Read the model definition and answer for the solid it produces. Units are mm, in the model's axes. Face numbers are marked on the shaded views. A direction names the side the tool comes from. Coordinates: 2 decimals unless noted, no trailing zeros. Loops run counter-clockwise (first coordinate to the right, second up) from the corner with the lowest first, then second, coordinate; pieces in that order, holes last.
from build123d import *

# Parameters (mm, degrees)
F0_R     = 12.7
F1_DEPTH = 25.4
F2_R     = 12.7
F3_DEPTH = 3.175
F5_DEPTH = 25.4


with BuildPart() as f1:
    # F0 (on Top) → F1 (new body)
    with BuildSketch(Plane.XY):
        Circle(F0_R)
        with BuildLine():
            ThreePointArc((8.614346, 1.798068), (8.753463, 0.903814), (8.8, 0))
            ThreePointArc((8.8, 0), (8.753463, -0.903814), (8.614346, -1.798068))
            Line((8.614346, -1.798068), (10.468267, -2.86843))
            Line((10.468267, -2.86843), (7.718267, -7.63157))
            Line((7.718267, -7.63157), (5.864346, -6.561208))
            ThreePointArc((5.864346, -6.561208), (4.4, -7.621024), (2.75, -8.359276))
            Line((2.75, -8.359276), (2.75, -10.5))
            Line((2.75, -10.5), (-2.75, -10.5))
            Line((-2.75, -10.5), (-2.75, -8.359276))
            ThreePointArc((-2.75, -8.359276), (-4.4, -7.621024), (-5.864346, -6.561208))
            Line((-5.864346, -6.561208), (-7.718267, -7.63157))
            Line((-7.718267, -7.63157), (-10.468267, -2.86843))
            Line((-10.468267, -2.86843), (-8.614346, -1.798068))
            ThreePointArc((-8.614346, -1.798068), (-8.8, 0), (-8.614346, 1.798068))
            Line((-8.614346, 1.798068), (-10.468267, 2.86843))
            Line((-10.468267, 2.86843), (-7.718267, 7.63157))
            Line((-7.718267, 7.63157), (-5.864346, 6.561208))
            ThreePointArc((-5.864346, 6.561208), (-4.4, 7.621024), (-2.75, 8.359276))
            Line((-2.75, 8.359276), (-2.75, 10.5))
            Line((-2.75, 10.5), (2.75, 10.5))
            Line((2.75, 10.5), (2.75, 8.359276))
            ThreePointArc((2.75, 8.359276), (4.4, 7.621024), (5.864346, 6.561208))
            Line((5.864346, 6.561208), (7.718267, 7.63157))
            Line((7.718267, 7.63157), (10.468267, 2.86843))
            Line((10.468267, 2.86843), (8.614346, 1.798068))
        make_face(mode=Mode.SUBTRACT)
    extrude(amount=F1_DEPTH)

    # F2 (on face) → F3 (join)
    with BuildSketch(Plane.XY.offset(25.4)):
        Circle(F2_R)
    extrude(amount=F3_DEPTH)

    # F4 (on face) → F5 (join)
    with BuildSketch(Plane.XY.offset(28.575)):
        Polygon((3.666174, 6.35), (-3.666174, 6.35), (-7.332348, 0), (-3.666174, -6.35), (3.666174, -6.35), (7.332348, 0), align=None)
    extrude(amount=F5_DEPTH)


solid = f1.part
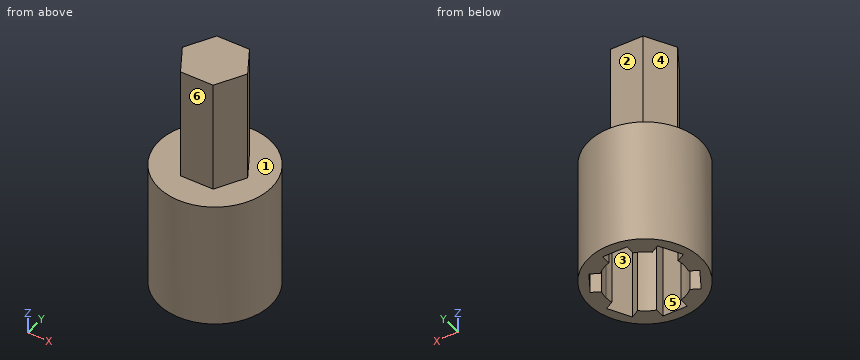
Q1. A cutting plane is placed at C-C (z = 49.5). Give the vertices of the cut face in (x, y), then the cut area to 3 significant figures.
Findings below:
outline: (-7.33, 0) - (-3.67, -6.35) - (3.67, -6.35) - (7.33, 0) - (3.67, 6.35) - (-3.67, 6.35) - close
area: 140 mm2
Q2. A cutting plane is placed at B-B (x = 0). Give the vertices of the cut face in (y, z) (3 decimals).
Findings below:
outline: (-12.7, 0) - (-10.5, 0) - (-10.5, 25.4) - (10.5, 25.4) - (10.5, 0) - (12.7, 0) - (12.7, 28.575) - (6.35, 28.575) - (6.35, 53.975) - (-6.35, 53.975) - (-6.35, 28.575) - (-12.7, 28.575) - close
Q3. Flat-ended cylindrical pins translate along their axes: pin 1 Ø12 at (x, y) = (1, 2.5) entering from -Z; pin 2 Ø0.6 at (y, z) = (-9.5, 10) entering from +X (3 decimals); pin 3 Ø1 at (x, z) = (5, 15.5) entering from -Y. Find the tip coordinate at first contact, or state that the pin passes through.
Findings below:
pin 1: stops at z = 25.4
pin 2: stops at x = 8.755
pin 3: stops at y = -11.88
Q4. Straight lines are drawn through the part: probe 1 along Z at (x, y) = (9, 1.75) (3 decimals); probe 2 along Z at (x, y) = (4.25, 6) (3 decimals); probe 3 along X at (y, z) = (8, 3.5). For each, find the intervals that lie inside material, in ascending order.
Findings below:
probe 1: z = 0 to 28.575
probe 2: z = 25.4 to 28.575
probe 3: x = -9.86 to -3.67, 3.67 to 9.86
Q5. Which of the six approach directions +Z, -Z, +X, -X, +Y, -Y give full straight-line access (tool end or side, diameter ignored) to the marked faces 4, 5 and 6?
Findings below:
face 4: +Z, -X, +Y
face 5: -Z
face 6: +Z, +X, -X, -Y
Q6. Determine the mould class of the marked faces 1, 2 and 3 for opening direction Y: +Y half, -Y half, draft (parallel to the pull), parting line (faces both ways), or undercut.
Findings below:
face 1: draft
face 2: +Y half
face 3: undercut
Q7. A cutting plane is placed at A-A (z = 7.5). Give the vertices of the cut face in (x, y), then the cut area to 3 significant figures.
Findings below:
outline: circle Ø25.4 at (0, 0); hole (-10.47, -2.87) - (-7.72, -7.63) - (-5.86, -6.56) arc R8.8 ccw to (-2.75, -8.36) - (-2.75, -10.5) - (2.75, -10.5) - (2.75, -8.36) arc R8.8 ccw to (5.86, -6.56) - (7.72, -7.63) - (10.47, -2.87) - (8.61, -1.8) arc R8.8 ccw to (8.8, 0) arc R8.8 ccw to (8.61, 1.8) - (10.47, 2.87) - (7.72, 7.63) - (5.86, 6.56) arc R8.8 ccw to (2.75, 8.36) - (2.75, 10.5) - (-2.75, 10.5) - (-2.75, 8.36) arc R8.8 ccw to (-5.86, 6.56) - (-7.72, 7.63) - (-10.47, 2.87) - (-8.61, 1.8) arc R8.8 ccw to (-8.61, -1.8) - close
area: 203 mm2
Q8. A cutting plane is placed at D-D (x = -4.5). Give the vertices of the cut face in (y, z) (3 decimals).
Findings below:
outline: (-11.876, 0) - (-7.562, 0) - (-7.562, 25.4) - (7.562, 25.4) - (7.562, 0) - (11.876, 0) - (11.876, 28.575) - (4.906, 28.575) - (4.906, 53.975) - (-4.906, 53.975) - (-4.906, 28.575) - (-11.876, 28.575) - close
